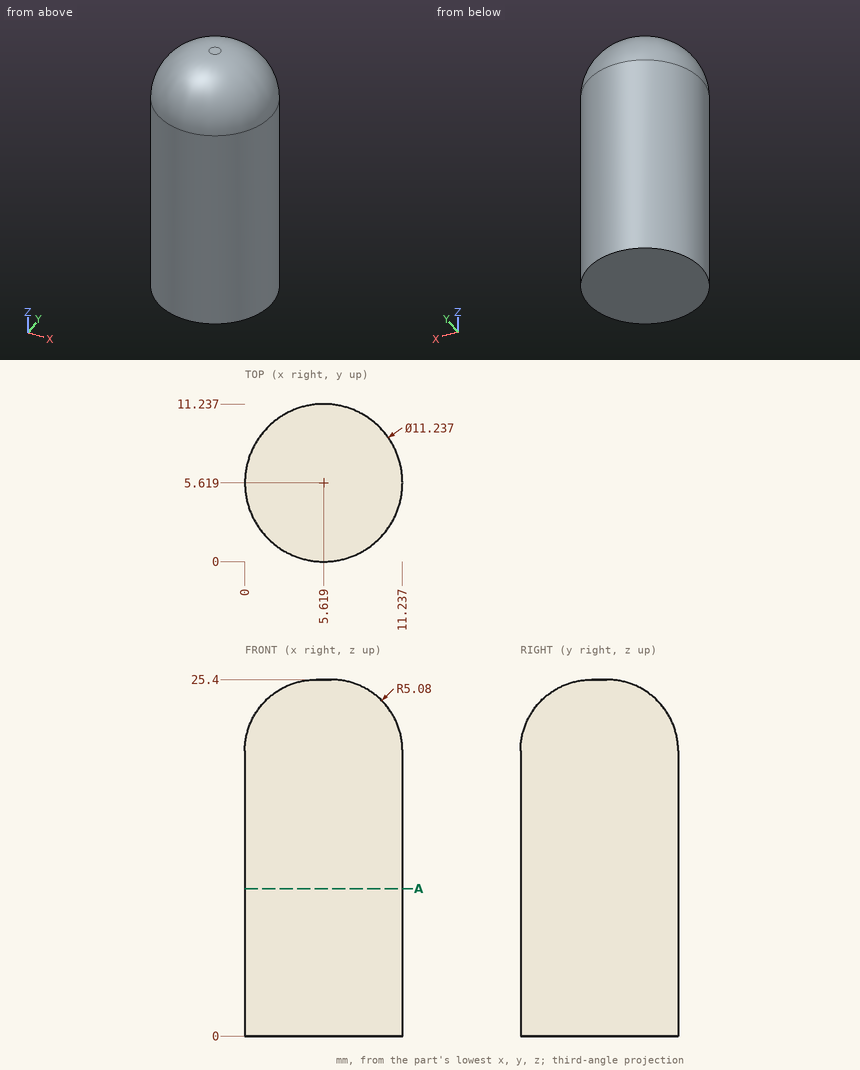
Input: dimensioned drawing with shaded views. Units: mm. Origin: part minimum x, y, z. Give positions to 0.01 mm unless a question says otherwise; leave off trailing zeros. Write each loop counter-clockwise with the first axis right and the second up, starting at its lowest first coordinate (ties: lowest second). Pieces come first, ordered by that corner, then holes.
1. Section query A-A, the plane z = 10.5. Return loops of the section in (x, y).
2. Pin query (flat end, axial travel): P1, Ø5, axis at x = 9.5, y = 4.5, coming from the +Z side; P2, Ø2, axis at x = 10, z = 10.5, coming from the +Y side (1 decimal); P3, Ø1, axis at x = 8, z = 8, coming from the +Y side. Return the tip coordinate at first contact, or that it passes through.
3. Line query: probe 1 along Z at (x, y) = (9.5, 4.5); probe 2 along Y at (x, z) = (4.25, 12); probe 3 along X at (y, z) = (2.5, 23.5) (1 decimal). Output: solid intervals per line, ascending.
Computed:
1. outline: circle Ø11.24 at (5.62, 5.62)
2. P1: stops at z = 25.3
2. P2: stops at y = 10.1
2. P3: stops at y = 10.91
3. probe 1: z = 0 to 24
3. probe 2: y = 0.17 to 11.07
3. probe 3: x = 2.4 to 8.9
